Can you work these out from the model? Positions are in its coordinate system, mm. A direction names the side the tool comes from. Give positions to 0.01 mm unless a question says otherwise; leave off trailing zeros. Use one line per item in the form item = value. Start each with the question number.
1. I need wall thicknesses on L1, parallel to Y at x = -23.98, z = 2; L2, parallel to X at y = 26.5, z = 8.5; L3, parallel to Y at x = 46, z = 8.25. Which ranges of each line are inside material? Lowest first, please.
2. I want a section at A-A, the plane z = 8.5. Count the separate pieces of the cut face and the enclosed holes in it, and give its area (3 significant figures).
3. Will these pins go through, and if not, where does the flat tip stop? P1, Ø2, axis at x = -36.5, y = 31.5, coming from the -Z side; P2, Ø6, axis at x = -24.5, z = 12, coming from the +Y side; P3, Ø3, axis at x = 24, z = 12, coming from the -Y side.
4. For faces 5 (the face through (17.77, -57.68, 23.99)), 6 (the face through (-23.716, 43.542, 3.451)), which set-ups out of +Z, -Z, +X, -X, +Y, -Y let a thin tool reach every point of the face, with its end or its side?
5. We'd pull the mould along Y, two halves only. Please class faces 1 (the face through (-55.1, -31.7, 24)), 2 (the face through (46.56, -15.035, 3.451)), 3 (the face through (18.559, 58.373, 11.339)), 4 (the face through (-25.9, -19.8, 19.9)): +Y half, -Y half, draft (parallel to the pull), parting line (faces both ways), or undercut.
```python
from build123d import *

# Parameters (mm, degrees)
SKETCH1_R           = 60
SKETCH1_R_2         = 2.55
SKETCH1_R_3         = 42.55
BOSS_EXTRUDE1_DEPTH = 25
BOSS_EXTRUDE2_START = -10
SKETCH3_R           = 42.55
SKETCH3_R_2         = 32.6
BOSS_EXTRUDE2_DEPTH = 10
BOSS_EXTRUDE3_DEPTH = 25
SKETCH8_R           = 5
CUT_EXTRUDE1_DEPTH  = 6
CHAMFER2_SIZE       = 0.5
CHAMFER3_SIZE       = 2
SKETCH9_R           = 2.025
CUT_EXTRUDE2_DEPTH  = 7


with BuildPart() as part:
    # Sketch1 → Boss-Extrude1 (new body)
    with BuildSketch(Plane.XY):
        Circle(SKETCH1_R)
        with Locations((0, 55)):
            Circle(SKETCH1_R_2, mode=Mode.SUBTRACT)
        with Locations((47.631397208, 27.5)):
            Circle(SKETCH1_R_2, mode=Mode.SUBTRACT)
        with Locations((47.631397208, -27.5)):
            Circle(SKETCH1_R_2, mode=Mode.SUBTRACT)
        with Locations((0, -55)):
            Circle(SKETCH1_R_2, mode=Mode.SUBTRACT)
        with Locations((-47.631397208, -27.5)):
            Circle(SKETCH1_R_2, mode=Mode.SUBTRACT)
        with Locations((-47.631397208, 27.5)):
            Circle(SKETCH1_R_2, mode=Mode.SUBTRACT)
        Circle(SKETCH1_R_3, mode=Mode.SUBTRACT)
    extrude(amount=BOSS_EXTRUDE1_DEPTH)

    # Sketch3 → Boss-Extrude2 (add)
    with BuildSketch(Plane.XY.offset(25).offset(BOSS_EXTRUDE2_START)):
        Circle(SKETCH3_R)
        Circle(SKETCH3_R_2, mode=Mode.SUBTRACT)
    extrude(amount=BOSS_EXTRUDE2_DEPTH)

    # Sketch7 → Boss-Extrude3 (add)
    with BuildSketch(Plane(origin=(0, 0, 0), x_dir=(-1, 0, 0), z_dir=(0, 0, -1))):
        with BuildLine():
            Line((-29.313322314, 52.351973553), (-7.5, 64.565857851))
            Line((-7.5, 64.565857851), (7.5, 64.565857851))
            Line((7.5, 64.565857851), (29.313322314, 52.351973553))
            ThreePointArc((29.313322314, 52.351973553), (0, 60), (-29.313322314, 52.351973553))
        make_face()
        with BuildLine():
            Line((59.665673116, 25.787738397), (59.994800192, 0.789904984))
            ThreePointArc((59.994800192, 0.789904984), (51.961524227, 30), (30.681477878, 51.56206857))
            Line((30.681477878, 51.56206857), (52.165673116, 38.778119454))
            Line((52.165673116, 38.778119454), (59.665673116, 25.787738397))
        make_face()
        with BuildLine():
            Line((52.165673116, -38.778119454), (30.681477878, -51.56206857))
            ThreePointArc((30.681477878, -51.56206857), (51.961524227, -30), (59.994800192, -0.789904984))
            Line((59.994800192, -0.789904984), (59.665673116, -25.787738397))
            Line((59.665673116, -25.787738397), (52.165673116, -38.778119454))
        make_face()
        with BuildLine():
            Line((-7.5, -64.565857851), (-29.313322314, -52.351973553))
            ThreePointArc((-29.313322314, -52.351973553), (0, -60), (29.313322314, -52.351973553))
            Line((29.313322314, -52.351973553), (7.5, -64.565857851))
            Line((7.5, -64.565857851), (-7.5, -64.565857851))
        make_face()
        with BuildLine():
            Line((-59.665673116, -25.787738397), (-59.994800192, -0.789904984))
            ThreePointArc((-59.994800192, -0.789904984), (-51.961524227, -30), (-30.681477878, -51.56206857))
            Line((-30.681477878, -51.56206857), (-52.165673116, -38.778119454))
            Line((-52.165673116, -38.778119454), (-59.665673116, -25.787738397))
        make_face()
        with BuildLine():
            Line((-52.165673116, 38.778119454), (-30.681477878, 51.56206857))
            ThreePointArc((-30.681477878, 51.56206857), (-51.961524227, 30), (-59.994800192, 0.789904984))
            Line((-59.994800192, 0.789904984), (-59.665673116, 25.787738397))
            Line((-59.665673116, 25.787738397), (-52.165673116, 38.778119454))
        make_face()
    extrude(amount=-BOSS_EXTRUDE3_DEPTH)

    # Sketch8 → Cut-Extrude1 (cut)
    with BuildSketch(Plane.XY.offset(25)):
        with Locations((0, 55)):
            Circle(SKETCH8_R)
        with Locations((47.631397208, 27.5)):
            Circle(SKETCH8_R)
        with Locations((47.631397208, -27.5)):
            Circle(SKETCH8_R)
        with Locations((0, -55)):
            Circle(SKETCH8_R)
        with Locations((-47.631397208, -27.5)):
            Circle(SKETCH8_R)
        with Locations((-47.631397208, 27.5)):
            Circle(SKETCH8_R)
    extrude(amount=-CUT_EXTRUDE1_DEPTH, mode=Mode.SUBTRACT)

    # Chamfer2
    chamfer2_edges = [part.edges().sort_by_distance(p)[0] for p in [
        (-32.6, 0, 15),
        (-32.6, 0, 25),
        (-42.55, 0, 0),
    ]]
    chamfer(chamfer2_edges, length=CHAMFER2_SIZE)

    # Chamfer3
    chamfer3_edges = [part.edges().sort_by_distance(p)[0] for p in [
        (-30, 51.961524227, 25),
        (-18.406661157, 58.458915702, 25),
        (0, 64.565857851, 25),
        (18.406661157, 58.458915702, 25),
        (-60, 0, 25),
        (-59.830236654, 13.28882169, 25),
        (-55.915673116, 32.282928925, 25),
        (-41.423575497, 45.170094012, 25),
        (-30, -51.961524227, 25),
        (-41.423575497, -45.170094012, 25),
        (-55.915673116, -32.282928925, 25),
        (-59.830236654, -13.28882169, 25),
        (30, -51.961524227, 25),
        (18.406661157, -58.458915702, 25),
        (0, -64.565857851, 25),
        (-18.406661157, -58.458915702, 25),
        (60, 0, 25),
        (59.830236654, -13.28882169, 25),
        (55.915673116, -32.282928925, 25),
        (41.423575497, -45.170094012, 25),
        (30, 51.961524227, 25),
        (41.423575497, 45.170094012, 25),
        (55.915673116, 32.282928925, 25),
        (59.830236654, 13.28882169, 25),
    ]]
    chamfer(chamfer3_edges, length=CHAMFER3_SIZE)

    # Sketch9 → Cut-Extrude2 (cut)
    with BuildSketch(Plane(origin=(0, 0, 0), x_dir=(-1, 0, 0), z_dir=(0, 0, -1))):
        with Locations((-8.328166601, 47.231379834)):
            Circle(SKETCH9_R)
        with Locations((8.328166601, 47.231379834)):
            Circle(SKETCH9_R)
        with Locations((23.98, 41.534578366)):
            Circle(SKETCH9_R)
        with Locations((36.739491492, 30.828093761)):
            Circle(SKETCH9_R)
        with Locations((45.067658093, 16.403286074)):
            Circle(SKETCH9_R)
        with Locations((47.96, 0)):
            Circle(SKETCH9_R)
        with Locations((45.067658093, -16.403286074)):
            Circle(SKETCH9_R)
        with Locations((36.739491492, -30.828093761)):
            Circle(SKETCH9_R)
        with Locations((23.98, -41.534578366)):
            Circle(SKETCH9_R)
        with Locations((8.328166601, -47.231379834)):
            Circle(SKETCH9_R)
        with Locations((-8.328166601, -47.231379834)):
            Circle(SKETCH9_R)
        with Locations((-23.98, -41.534578366)):
            Circle(SKETCH9_R)
        with Locations((-36.739491492, -30.828093761)):
            Circle(SKETCH9_R)
        with Locations((-45.067658093, -16.403286074)):
            Circle(SKETCH9_R)
        with Locations((-47.96, 0)):
            Circle(SKETCH9_R)
        with Locations((-45.067658093, 16.403286074)):
            Circle(SKETCH9_R)
        with Locations((-36.739491492, 30.828093761)):
            Circle(SKETCH9_R)
        with Locations((-23.98, 41.534578366)):
            Circle(SKETCH9_R)
    extrude(amount=-CUT_EXTRUDE2_DEPTH, mode=Mode.SUBTRACT)


solid = part.part
```
Check result:
q1.L1 = -55.34 to -43.56, -39.51 to -35.15, 35.15 to 39.51, 43.56 to 55.34
q1.L2 = -59.25 to -49.98, -45.29 to -33.29, 33.29 to 45.29, 49.98 to 59.25
q1.L3 = -42.45 to -29.46, -25.54 to 25.54, 29.46 to 42.45
q2.separate_pieces = 1
q2.enclosed_holes = 7
q2.area = 6,380 mm2
q3.P1 = 7
q3.P2 = 56.73
q3.P3 = -56.17
q4.face_5 = +Z, +X, -Y
q4.face_6 = -Z
q5.face_1 = -Y half
q5.face_2 = undercut
q5.face_3 = +Y half
q5.face_4 = undercut
